Design review of the part built by this model. Coordinates are the model's own, in mm. Give positions to 0.01 mm unless a question says otherwise; leave off trailing zeros. Loops run counter-clockwise (first coordinate to the right, second up) from the corner with the lowest first, then second, coordinate; pieces in that order, holes last. Notation, with made-up numbers: (-34, 51.25) -> (-21, 51.25) arc R10 ccw to (-21, 66.25) -> close; hole circle Ø10 at (39, -13). An arc over 180 degrees is marked (long way). Use a Markdown table: item, result. Add a question column.
1. Add section D-D (z = -7). State the section outline as (x, y) points, and give its area (3 significant figures).
2. Draft analysis for pull direction X (two halves, no side actions). For faces 1 (the flat face through (4, 0, 24)), 2 (the flat face through (21.59, -3, 30)), 3 (the cylindrical face through (14.47, -3.13, 2.39)), state which applies: pulls with the +X half, pulls with the -X half, needs draft (parallel to the pull), parting line crosses it, or undercut.
3. To check wall thickness, follow line 1 (Z direction, x = -9.5, y = -4.75); line 2 (Z direction, x = -1, y = -2.75); line 3 (X direction, y = -2, z = 1). State the ranges of each line that lie inside material, in increasing order.
4. Add section A-A (x = 8.5). State the section outline as (y, z) points.
5. Add section B-B (y = -2.25). Count the separate pieces of the cut face and the enclosed holes in it, and give its area (3 significant figures).
6. For pin 1 Ø2 at (x, y) = (0, -0.5) entering from -Z; pin 2 Ø4 at (x, z) = (13, 3) entering from -Y; pin 3 Ø3 at (x, y) = (16.5, -1) entering from +Z; pin 4 Ø3 at (x, y) = (16.5, -5) entering from -Z, all flat-tipped, find the tip position at first contact; note any pin that passes through.
7. Add section C-C (x = -1.5). State the section outline as (y, z) points, and give its area (3 significant figures).
```python
from build123d import *

# Parameters (mm, degrees)
F0_R     = 4.7625
F0_R_2   = 3.175
F0_R_3   = 1.5875
F0_R_4   = 3.96875
F1_DEPTH = 6.35


with BuildPart() as f1:
    # F0 (on Front) → F1 (new body)
    with BuildSketch(Plane.XZ):
        Polygon((-13.97, 61.09232), (-13.97, -15.10768), (-7.2898, -15.10768), (21.59, 0), (21.59, 60.86069), align=None)
        Circle(F0_R, mode=Mode.SUBTRACT)
        with Locations((-7.1628, 11.049)):
            Circle(F0_R_2, mode=Mode.SUBTRACT)
        with Locations((13.0048, 2.9972)):
            Circle(F0_R_3, mode=Mode.SUBTRACT)
        with Locations((6.985, 11.557)):
            Circle(F0_R_4, mode=Mode.SUBTRACT)
        with Locations((-7.1628, 36.957)):
            Circle(F0_R_2, mode=Mode.SUBTRACT)
        with Locations((0, 48.006)):
            Circle(F0_R, mode=Mode.SUBTRACT)
        with Locations((6.1976, 36.3728)):
            Circle(F0_R_2, mode=Mode.SUBTRACT)
    extrude(amount=F1_DEPTH)


solid = f1.part
```
Taken from the geometry:
| question | item | result |
|---|---|---|
| 1 | outline | (-13.97, -6.35) -> (8.21, -6.35) -> (8.21, 0) -> (-13.97, 0) -> close |
| 1 | area | 141 mm^2 |
| 2 | face 1 | needs draft |
| 2 | face 2 | pulls with the +X half |
| 2 | face 3 | undercut |
| 3 | line 1 | z = -15.11 to 8.9, 13.2 to 34.81, 39.11 to 61.06 |
| 3 | line 2 | z = -11.82 to -4.66, 4.66 to 43.35, 52.66 to 61.01 |
| 3 | line 3 | x = -13.97 to -4.66, 4.66 to 21.59 |
| 4 | outline | (-6.35, -6.85) -> (0, -6.85) -> (0, 7.89) -> (-6.35, 7.89) -> close; (-6.35, 15.23) -> (0, 15.23) -> (0, 34.19) -> (-6.35, 34.19) -> close; (-6.35, 38.56) -> (0, 38.56) -> (0, 60.95) -> (-6.35, 60.95) -> close |
| 5 | separate pieces | 1 |
| 5 | enclosed holes | 7 |
| 5 | area | 2,190 mm^2 |
| 6 | pin 1 | stops at z = -11.82 |
| 6 | pin 2 | stops at y = -6.35 |
| 6 | pin 3 | stops at z = 60.9 |
| 6 | pin 4 | stops at z = -3.45 |
| 7 | outline | (-6.35, -12.08) -> (0, -12.08) -> (0, -4.52) -> (-6.35, -4.52) -> close; (-6.35, 4.52) -> (0, 4.52) -> (0, 43.49) -> (-6.35, 43.49) -> close; (-6.35, 52.53) -> (0, 52.53) -> (0, 61.01) -> (-6.35, 61.01) -> close |
| 7 | area | 349 mm^2 |
